Design review of the part built by this model. Coordinates are the model's own, in mm. Coordinates: 2 decimals unless noted, no trailing zeros. Loops run counter-clockwise (first coordinate to the right, second up) from the corner with the lowest first, then second, coordinate; pieces in that order, holes last. Notation, with made-up numbers: (59, 35.5) -> (102, 35.5) arc R29 cw to (102, 74.5) -> close; hole circle Ø10 at (-16, -26). An arc over 180 degrees is marked (long way). Use CSV: the item, a comma, the result in double quotes.
```python
from build123d import *

# Parameters (mm, degrees)
CROQUIS1_W              = 15
CROQUIS1_H              = 15
CROQUIS1_R              = 1.6
SALIENTE_EXTRUIR1_DEPTH = 3
CORTAR_EXTRUIR1_DEPTH   = 2.3
CROQUIS3_W              = 15
CROQUIS3_H              = 15
CROQUIS3_R              = 1.6
SALIENTE_EXTRUIR2_DEPTH = 1


with BuildPart() as part:
    # Croquis1 → Saliente-Extruir1 (new body)
    with BuildSketch(Plane(origin=(0, 0, 0), x_dir=(1, 0, 0), z_dir=(0, 1, 0))):
        with Locations((7.5, 7.5)):
            Rectangle(CROQUIS1_W, CROQUIS1_H)
        with Locations(Location((7.5, 7.5, 0), (0, 0, 270))):
            Circle(CROQUIS1_R, mode=Mode.SUBTRACT)
    extrude(amount=SALIENTE_EXTRUIR1_DEPTH)

    # Croquis2 → Cortar-Extruir1 (cut)
    with BuildSketch(Plane(origin=(0, 3, 0), x_dir=(1, 0, 0), z_dir=(0, 1, 0))):
        Polygon((7.5, 4.324573519), (10.25, 5.91228676), (10.25, 9.08771324), (7.5, 10.675426481), (4.75, 9.08771324), (4.75, 5.91228676), align=None)
    extrude(amount=-CORTAR_EXTRUIR1_DEPTH, mode=Mode.SUBTRACT)

    # Croquis3 → Saliente-Extruir2 (add)
    with BuildSketch(Plane(origin=(0, 3, 0), x_dir=(1, 0, 0), z_dir=(0, 1, 0))):
        with Locations((7.5, 7.5)):
            Rectangle(CROQUIS3_W, CROQUIS3_H)
        with Locations(Location((7.5, 7.5, 0), (0, 0, 270))):
            Circle(CROQUIS3_R, mode=Mode.SUBTRACT)
    extrude(amount=SALIENTE_EXTRUIR2_DEPTH)


solid = part.part
```
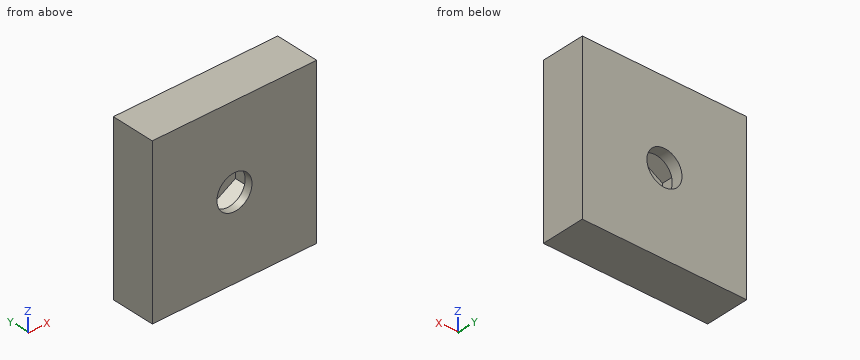
Item 1: Add section C-C (x = 5.5). Give the boundary of the cut face in (y, z), then the cut area to 3 significant figures.
Checked values:
outline,"(0, -15) -> (4, -15) -> (4, 0) -> (0, 0) -> close; hole (0.7, -9.52) -> (3, -9.52) -> (3, -5.48) -> (0.7, -5.48) -> close"
area,"50.7 mm^2"
Item 2: Add section D-D (z = -5.25). Give the boundary of the cut face in (x, y), then the cut area to 3 significant figures.
Checked values:
outline,"(0, 0) -> (15, 0) -> (15, 4) -> (0, 4) -> close; hole (5.9, 0.7) -> (9.1, 0.7) -> (9.1, 3) -> (5.9, 3) -> close"
area,"52.6 mm^2"
Item 3: To check wall thickness, follow line 1 along Z through (x, y) = (7.5, 0.5); line 2 along X through (y, z) = (1.7, -5.25); line 3 along Y through (x, z) = (5.5, -8.5). State the ranges of each line that lie inside material, in increasing order.
Checked values:
line 1,"-15 to -9.1, -5.9 to 0"
line 2,"0 to 5.9, 9.1 to 15"
line 3,"0 to 0.7, 3 to 4"
Item 4: Add section A-A (y = 1.5). Give the boundary of the cut face in (x, z).
Checked values:
outline,"(0, -15) -> (15, -15) -> (15, 0) -> (0, 0) -> close; hole (4.75, -9.09) -> (7.5, -10.68) -> (10.25, -9.09) -> (10.25, -5.91) -> (7.5, -4.32) -> (4.75, -5.91) -> close"
Item 5: Add section B-B (z = -7.5). Give the boundary of the cut face in (x, y), then the cut area to 3 significant figures.
Checked values:
outline,"(0, 0) -> (5.9, 0) -> (5.9, 0.7) -> (4.75, 0.7) -> (4.75, 3) -> (5.9, 3) -> (5.9, 4) -> (0, 4) -> close; (9.1, 0) -> (15, 0) -> (15, 4) -> (9.1, 4) -> (9.1, 3) -> (10.25, 3) -> (10.25, 0.7) -> (9.1, 0.7) -> close"
area,"41.9 mm^2"
